```python
from build123d import *

# Parameters (mm, degrees)
SKETCH_1_R      = 1.5
SKETCH_1_R_2    = 8
EXTRUDE_1_DEPTH = 2
SKETCH_3_R      = 10
SKETCH_3_R_2    = 8
EXTRUDE_2_DEPTH = 10


with BuildPart() as part:
    # 草图1 → 凸台-拉伸1 (new body)
    with BuildSketch(Plane.XY):
        with BuildLine():
            Line((17.5, 16.5), (-17.5, 16.5))
            Line((-17.5, 16.5), (-17.5, 10.5))
            ThreePointArc((-17.5, 10.5), (-11.309475019, 0), (-17.5, -10.5))
            Line((-17.5, -10.5), (-17.5, -16.5))
            Line((-17.5, -16.5), (17.5, -16.5))
            Line((17.5, -16.5), (17.5, -10.5))
            ThreePointArc((17.5, -10.5), (11.309475019, 0), (17.5, 10.5))
            Line((17.5, 10.5), (17.5, 16.5))
        make_face()
        with Locations((-13.5, -12.5)):
            Circle(SKETCH_1_R, mode=Mode.SUBTRACT)
        with Locations((13.5, -12.5)):
            Circle(SKETCH_1_R, mode=Mode.SUBTRACT)
        Circle(SKETCH_1_R_2, mode=Mode.SUBTRACT)
        with Locations((-13.5, 12.5)):
            Circle(SKETCH_1_R, mode=Mode.SUBTRACT)
        with Locations((13.5, 12.5)):
            Circle(SKETCH_1_R, mode=Mode.SUBTRACT)
    extrude(amount=EXTRUDE_1_DEPTH)

    # 草图3 → 凸台-拉伸2 (add)
    with BuildSketch(Plane.XY.offset(2)):
        Circle(SKETCH_3_R)
        Circle(SKETCH_3_R_2, mode=Mode.SUBTRACT)
    extrude(amount=EXTRUDE_2_DEPTH)


solid = part.part
```
The listing builds one solid part. Answer for the finished solid, in the listing's coordinates (mm). A direction names the side the tool comes from. Give positions to 0.01 mm unless a question says otherwise; leave off trailing zeros. Order: outer loops, then holes, each group sorted by start corner. A loop starts at its lowest first (then second) coordinate and runs counter-clockwise, first axis right, second up. Notation, with made-up numbers: M 83,30.25 L 111,30.25 A14 cw 111,49.25 Z; hole C -30,63.25 d2. An arc over 180 degrees is marked long. Put each result on its own line as item: value. Start each with the question number.
Item 1: The part is cut by section C-C, the plane y = -12.5. Determine the outline of the cut face in (x, z), and give its area (3 significant figures).
Item 2: The part is cut by section D-D, the plane z = 1. Determine the outline of the cut face in (x, y), and give its area (3 significant figures).
Item 3: The part is cut by section A-A, the plane y = 0. Determine the outline of the cut face in (x, z).
Item 4: The part is cut by section B-B, the plane x = 0. Determine the outline of the cut face in (y, z).
Item 5: For a pull along Y with two mould halves and no side action, classify faces 3 (the face through (0, 16.5, 1)), 4 (the face through (12, -12.43, 0.99)), 5 (the face through (-11.31, 0.18, 0.99)), 6 (the face through (-17.5, 14, 1)) as +Y half, -Y half, draft (parallel to the pull), parting line (faces both ways), or undercut.
Item 6: Which of the six approach directions +Z, -Z, +X, -X, +Y, -Y give full straight-line access (tool end or side, diameter ignored) to faces 1 (the face through (-2.17, -9.76, 6.93)), 2 (the face through (0, -16.5, 1))?
Item 7: Find the intervals of material crossed by line 1 along Y through (x, z) = (-13.5, 1.15); line 2 along Y through (x, z) = (0, 7); line 3 along Z through (x, y) = (8.5, 14.5), in increasing order.
Item 8: Flat-ended cylindrical pins translate along their axes: P1, Ø4, axis at y = 0, z = 8.5, coming from the +X side; P2, Ø2, axis at x = 1, z = 4, coming from the +Y side; P3, Ø3.5, axis at x = -13.5, y = -12.5, coming from the +Z side; P4, Ø13, axis at x = 0, y = 0, coming from the +Z side. Find the tip coordinate at first contact, or state that the pin passes through.
Answer key:
1. outline: M -17.5,0 L -15,0 L -15,2 L -17.5,2 Z; M -12,0 L 12,0 L 12,2 L -12,2 Z; M 15,0 L 17.5,0 L 17.5,2 L 15,2 Z
1. area: 58.0 mm²
2. outline: M -17.5,-16.5 L 17.5,-16.5 L 17.5,-10.5 A12 cw 17.5,10.5 L 17.5,16.5 L -17.5,16.5 L -17.5,10.5 A12 cw -17.5,-10.5 Z; hole C -13.5,-12.5 d3; hole C -13.5,12.5 d3; hole C 0,0 d16; hole C 13.5,-12.5 d3; hole C 13.5,12.5 d3
2. area: 741 mm²
3. outline: M -11.31,0 L -8,0 L -8,12 L -10,12 L -10,2 L -11.31,2 Z; M 8,0 L 11.31,0 L 11.31,2 L 10,2 L 10,12 L 8,12 Z
4. outline: M -16.5,0 L -8,0 L -8,12 L -10,12 L -10,2 L -16.5,2 Z; M 8,0 L 16.5,0 L 16.5,2 L 10,2 L 10,12 L 8,12 Z
5. face 3: +Y half
5. face 4: undercut
5. face 5: undercut
5. face 6: draft
6. face 1: +Z
6. face 2: +Z, -Z, +X, -X, -Y
7. line 1: y = -16.5 to -14, -11 to -6.91, 6.91 to 11, 14 to 16.5
7. line 2: y = -10 to -8, 8 to 10
7. line 3: z = 0 to 2
8. P1: stops at x = 10
8. P2: stops at y = 10
8. P3: stops at z = 2
8. P4: passes through
